```python
from build123d import *

# Parameters (mm, degrees)
BOSS_EXTRUDE1_DEPTH = 3
BOSS_EXTRUDE2_DEPTH = 15
BOSS_EXTRUDE3_DEPTH = 42
SKETCH6_W           = 2.622655796
SKETCH6_H           = 42
SKETCH6_H_2         = 45
BOSS_EXTRUDE4_DEPTH = 4
CUT_EXTRUDE1_DEPTH  = 88.488342941


with BuildPart() as part:
    # Sketch1 → Boss-Extrude1 (new body)
    with BuildSketch(Plane(origin=(0, 0, 0), x_dir=(1, 0, 0), z_dir=(0, 1, 0))):
        Polygon((-60, 0), (0, 0), (0, 24), (-60, 15), align=None)
        Polygon((-60, -15), (0, -24), (0, 0), (-60, 0), align=None)
    extrude(amount=BOSS_EXTRUDE1_DEPTH)

    # Sketch3 → Boss-Extrude2 (add, symmetric)
    with BuildSketch(Plane.XY):
        Polygon((-64.095320817, 45), (-61.082922988, 45), (-56.987602171, 0), (-60, 0), align=None)
    extrude(amount=BOSS_EXTRUDE2_DEPTH, both=True)

    # Sketch4 → Boss-Extrude3 (add)
    with BuildSketch(Plane(origin=(0, 3, 0), x_dir=(1, 0, 0), z_dir=(0, 1, 0))):
        Polygon((-57.260623559, 12.377344204), (0, 20.966437738), (0, 24), (-60, 15), (-57.260623559, 15), align=None)
        Polygon((0, -24), (0, -20.966437738), (-57.260623559, -12.377344204), (-57.260623559, -15), (-60, -15), align=None)
    extrude(amount=BOSS_EXTRUDE3_DEPTH)

    # Sketch6 → Boss-Extrude4 (add)
    with BuildSketch(Plane.ZY.offset(57.260623559)):
        with Locations((-13.688672102, 24)):
            Rectangle(SKETCH6_W, SKETCH6_H)
        with Locations((13.688672102, 22.5)):
            Rectangle(SKETCH6_W, SKETCH6_H_2)
    extrude(amount=BOSS_EXTRUDE4_DEPTH)

    # Sketch7 → Cut-Extrude1 (cut, through all)
    with BuildSketch(Plane.XY.offset(15)):
        Polygon((-61.260623559, 13.851920935), (-60, 0), (-61.260623559, 0), align=None)
    extrude(amount=-CUT_EXTRUDE1_DEPTH, mode=Mode.SUBTRACT)


solid = part.part
```
Read the model definition and answer for the solid it produces. Units are mm, in the model's axes. A direction names the side the tool comes from. Round coordinates to 2 decimals unless told otherwise and drop trailing zeros. Write each loop counter-clockwise with the first axis right and the second up, starting at its lowest first coordinate (ties: lowest second). Pieces come first, ordered by that corner, then holes. Notation, with made-up numbers: M -26.75,-31 L -9.75,-31 A34 ccw -9.75,2 Z; hole C 42,42.25 d2. An arc over 180 degrees is marked long. One line per item, written item: value.
Q1. Which of the six approach directions +Z, -Z, +X, -X, +Y, -Y give full straight-line access (tool end or side, diameter ignored) to faces 1 (the flat face through (-62, 28, -15)), 2 (the flat face through (0, 2, 4)), 3 (the flat face through (-62, 28, 15)), 4 (the flat face through (-37, 45, -16)), 5 (the flat face through (-59.2, 24.3, 0.2))?
Data:
face 1: -Z, -X, +Y, -Y
face 2: +Z, -Z, +X, +Y, -Y
face 3: +Z, -X, +Y, -Y
face 4: +Z, -Z, +X, -X, +Y
face 5: +X, +Y
Q2. Find section C-C on x = -30. Write down the section's boundary in (y, z), plus the area to 3 significant figures.
Data:
outline: M 0,-19.5 L 45,-19.5 L 45,-16.47 L 3,-16.47 L 3,16.47 L 45,16.47 L 45,19.5 L 0,19.5 Z
area: 372 mm2
Q3. Find section B-B on y = 19.5. Write down the section's boundary in (x, z), plus the area to 3 significant figures.
Data:
outline: M -61.77,-15 L -60,-15 L 0,-24 L 0,-20.97 L -57.26,-12.38 L -58.76,-12.38 L -58.76,12.38 L -57.26,12.38 L 0,20.97 L 0,24 L -60,15 L -61.77,15 Z
area: 447 mm2
Q4. Find section D-D on y = 7.5. Write down the section's boundary in (x, z), plus the area to 3 significant figures.
Data:
outline: M -60.68,-15 L -60,-15 L 0,-24 L 0,-20.97 L -57.26,-12.38 L -57.67,-12.38 L -57.67,12.38 L -57.26,12.38 L 0,20.97 L 0,24 L -60,15 L -60.68,15 Z
area: 441 mm2
Q5. Find section A-A on z = -3. Write down the section's boundary in (x, y), plus the area to 3 significant figures.
Data:
outline: M -64.1,45 L -60,0 L 0,0 L 0,3 L -57.26,3 L -61.08,45 Z
area: 307 mm2
Q6. Flat-ended cylindrical pins translate along their axes: pin 1 Ø3.5 at (x, y) = (-62.5, 20) entering from +Z; pin 2 Ø4 at (x, y) = (-59.5, 24) entering from -Z (3 decimals); pin 3 Ø1.1 at (x, y) = (-59, 21) entering from +Z. Find the tip coordinate at first contact, or state that the pin passes through.
Data:
pin 1: z = 15
pin 2: z = -15.375
pin 3: z = 15.23
Q7. Straight lines are drawn through the part: line 1 (Y direction, x = -5, z = 3); line 2 (Z direction, x = -13.5, y = 34.5) (3 decimals); line 3 (Z direction, x = -54.5, y = 16.5) (3 decimals). For each, find the intervals that lie inside material, in ascending order. Write a range as [from, to].
Data:
line 1: [0, 3]
line 2: [-21.975, -18.941], [18.941, 21.975]
line 3: [-15.825, -12.791], [12.791, 15.825]
Q8. For a pull along Z with two mould halves and no side action, classify faces 6 (the flat face through (-30, 0, 0)), 7 (the flat face through (-58, 33, 12.377)), 8 (the flat face through (-29.58, 22.185, -19.563)) as +Z half, -Z half, draft (parallel to the pull), parting line (faces both ways), or undercut.
Data:
face 6: draft
face 7: undercut
face 8: -Z half
